Verification items for the finished model (mm, model axes). Face numbers are marked on the shaded views. A direction names the side the tool comes from. Round coordinates to 2 decimals unless told otherwise and drop trailing zeros. Write each loop counter-clockwise with the first axis right and the second up, starting at its lowest first coordinate (ties: lowest second). Pieces come first, ordered by that corner, then holes. Notation, with made-up numbers: (-19, 15.5) - (-3, 15.5) arc R15 ccw to (-3, 21.5) - close; hole circle Ø8 at (49, 11.25). An arc over 180 degrees is marked (long way). Write each question's results on one line, items separated by ' | '.
```python
from build123d import *

# Parameters (mm, degrees)
SKETCH1_W            = 600
SKETCH1_H            = 350
SKETCH1_W_2          = 500
SKETCH1_H_2          = 250
BOSS_EXTRUDE1_DEPTH  = 25
SKETCH2_W            = 50
SKETCH2_H            = 50
BOSS_EXTRUDE2_DEPTH  = 350
SKETCH6_W            = 50
SKETCH6_H            = 25
BOSS_EXTRUDE5_DEPTH  = 300
SKETCH7_W            = 50
SKETCH7_H            = 50
BOSS_EXTRUDE6_DEPTH  = 300
SKETCH8_W            = 50
SKETCH8_H            = 50
BOSS_EXTRUDE7_DEPTH  = 50
SKETCH9_W            = 333.649864746
SKETCH9_H            = 350
SKETCH9_W_2          = 233.483328298
SKETCH9_H_2          = 250
BOSS_EXTRUDE8_DEPTH  = 50
SKETCH10_W           = 50
SKETCH10_H           = 50
BOSS_EXTRUDE10_DEPTH = 10
BOSS_EXTRUDE13_DEPTH = 50
SKETCH15_W           = 30
SKETCH15_H           = 40
CUT_EXTRUDE1_DEPTH   = 50
SKETCH16_R           = 12
CUT_EXTRUDE2_DEPTH   = 50
SKETCH17_W           = 49.023713481
SKETCH17_H           = 36.523713481
CUT_EXTRUDE3_DEPTH   = 100
SKETCH18_W           = 57.595301864
SKETCH18_H           = 39.795828349
CUT_EXTRUDE4_DEPTH   = 100


with BuildPart() as part:
    # Sketch1 → Boss-Extrude1 (new body)
    with BuildSketch(Plane.XY):
        with Locations((250, 125)):
            Rectangle(SKETCH1_W, SKETCH1_H)
        with Locations((250, 125)):
            Rectangle(SKETCH1_W_2, SKETCH1_H_2, mode=Mode.SUBTRACT)
    extrude(amount=BOSS_EXTRUDE1_DEPTH)

    # Sketch2 → Boss-Extrude2 (add)
    with BuildSketch(Plane.XY.offset(25)):
        with Locations((-25, 275)):
            Rectangle(SKETCH2_W, SKETCH2_H)
        with Locations((-25, -25)):
            Rectangle(SKETCH2_W, SKETCH2_H)
    extrude(amount=BOSS_EXTRUDE2_DEPTH)

    # Sketch6 → Boss-Extrude5 (add)
    with BuildSketch(Plane.XZ.offset(-250)):
        with Locations((258.483328298, 12.5)):
            Rectangle(SKETCH6_W, SKETCH6_H)
    extrude(amount=BOSS_EXTRUDE5_DEPTH)

    # Sketch7 → Boss-Extrude6 (add)
    with BuildSketch(Plane.XY.offset(25)):
        with Locations((258.483328298, 119.33659126)):
            Rectangle(SKETCH7_W, SKETCH7_H)
    extrude(amount=BOSS_EXTRUDE6_DEPTH)

    # Sketch8 → Boss-Extrude7 (add)
    with BuildSketch(Plane.XY.offset(325)):
        with Locations((258.483328298, 119.33659126)):
            Rectangle(SKETCH8_W, SKETCH8_H)
    extrude(amount=BOSS_EXTRUDE7_DEPTH)

    # Sketch9 → Boss-Extrude8 (add)
    with BuildSketch(Plane.XY.offset(375)):
        with Locations((116.824932373, 125)):
            Rectangle(SKETCH9_W, SKETCH9_H)
        with Locations((116.741664149, 125)):
            Rectangle(SKETCH9_W_2, SKETCH9_H_2, mode=Mode.SUBTRACT)
    extrude(amount=-BOSS_EXTRUDE8_DEPTH)

    # Sketch10 → Boss-Extrude10 (add)
    with BuildSketch(Plane(origin=(283.483328298, 0, 0), x_dir=(0, 0, -1), z_dir=(1, 0, 0))):
        with Locations((-175, 119.33659126)):
            Rectangle(SKETCH10_W, SKETCH10_H)
    extrude(amount=BOSS_EXTRUDE10_DEPTH)

    # Sketch12 → Boss-Extrude13 (add)
    with BuildSketch(Plane.XZ.offset(-94.33659126)):
        with BuildLine():
            Line((293.483328298, 150), (323.483328298, 150))
            ThreePointArc((323.483328298, 150), (337.625463922, 155.857864376), (343.483328298, 170))
            Line((343.483328298, 170), (343.483328298, 180))
            ThreePointArc((343.483328298, 180), (337.625463922, 194.142135624), (323.483328298, 200))
            Line((323.483328298, 200), (293.483328298, 200))
            Line((293.483328298, 200), (293.483328298, 150))
        make_face()
    extrude(amount=-BOSS_EXTRUDE13_DEPTH)

    # Sketch15 → Cut-Extrude1 (cut)
    with BuildSketch(Plane.XY.offset(200)):
        with Locations((303.483328298, 119.33659126)):
            Rectangle(SKETCH15_W, SKETCH15_H)
    extrude(amount=-CUT_EXTRUDE1_DEPTH, mode=Mode.SUBTRACT)

    # Sketch16 → Cut-Extrude2 (cut)
    with BuildSketch(Plane.XZ.offset(-94.33659126)):
        with Locations(Location((323.483328298, 175, 0), (0, 0, 270))):
            Circle(SKETCH16_R)
    extrude(amount=-CUT_EXTRUDE2_DEPTH, mode=Mode.SUBTRACT)

    # Sketch17 → Cut-Extrude3 (cut)
    with BuildSketch(Plane(origin=(288.483328298, 0, 0), x_dir=(0, 0, -1), z_dir=(1, 0, 0))):
        with Locations((-175.48814326, 119.782326646)):
            Rectangle(SKETCH17_W, SKETCH17_H)
    extrude(amount=CUT_EXTRUDE3_DEPTH, mode=Mode.SUBTRACT)

    # Sketch18 → Cut-Extrude4 (cut)
    with BuildSketch(Plane.XY.offset(200)):
        with Locations((317.28097923, 119.438677086)):
            Rectangle(SKETCH18_W, SKETCH18_H)
    extrude(amount=-CUT_EXTRUDE4_DEPTH, mode=Mode.SUBTRACT)


solid = part.part
```
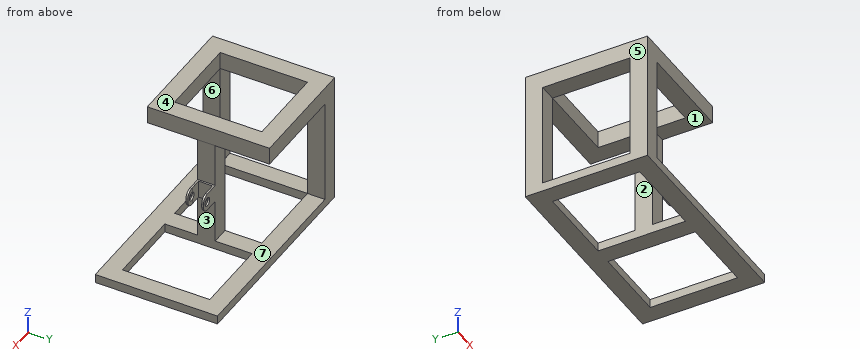
(1) Thickness scan on L1, parallel to Z at x = 254, y = 246.5; L2, parallel to X at y = 141.55, z = 175; L3, parallel to Y at x = 48.5, z = 335.5. Record the ranges inside material, lowest first.
Answer:
L1: 0 to 25, 325 to 375 | L2: 233.48 to 311.48, 335.48 to 343.48 | L3: -50 to 0, 250 to 300
(2) Section check B-B (z = 247.5). Record the cut outline in (x, y), plus the area to 3 significant figures.
Answer:
outline: (-50, -50) - (0, -50) - (0, 0) - (-50, 0) - close; (-50, 250) - (0, 250) - (0, 300) - (-50, 300) - close; (233.48, 94.34) - (283.48, 94.34) - (283.48, 144.34) - (233.48, 144.34) - close | area: 7,500 mm2
(3) Section check A-A (x = 130.5). Record the cut outline in (y, z).
Answer:
outline: (-50, 0) - (0, 0) - (0, 25) - (-50, 25) - close; (-50, 325) - (0, 325) - (0, 375) - (-50, 375) - close; (250, 0) - (300, 0) - (300, 25) - (250, 25) - close; (250, 325) - (300, 325) - (300, 375) - (250, 375) - close
(4) Set-up check for the marked faces 4, 5, 6 and 7: record each of +Z, -Z, +X, -X, +Y, -Y from which the full face is reachable in a straight line by a thin tool's end or side.
Answer:
face 4: +Z, +X, -X, +Y, -Y | face 5: +Z, -Z, -X, +Y, -Y | face 6: +X, +Y, -Y | face 7: +X
(5) Section check D-D (x = 372). Record the cut outline in (y, z).
Answer:
outline: (-50, 0) - (0, 0) - (0, 25) - (-50, 25) - close; (250, 0) - (300, 0) - (300, 25) - (250, 25) - close
(6) Go/stop test with flat-tipped pins: pin 1 Ø15 at (y, z) = (160, 345.5) entering from +X; pin 2 Ø6 at (x, y) = (303, 143.5) entering from +Z; pin 3 Ø3 at (y, z) = (118.5, 84) entering from -X. Record where each tip stops, or that it passes through.
Answer:
pin 1: x = 283.65 | pin 2: z = 200 | pin 3: x = 233.48
(7) Section check C-C (y = 45). Record the cut outline in (x, z).
Answer:
outline: (-50, 0) - (0, 0) - (0, 25) - (-50, 25) - close; (-50, 325) - (0, 325) - (0, 375) - (-50, 375) - close; (233.48, 0) - (283.48, 0) - (283.48, 25) - (233.48, 25) - close; (233.48, 325) - (283.65, 325) - (283.65, 375) - (233.48, 375) - close; (500, 0) - (550, 0) - (550, 25) - (500, 25) - close
(8) Mould release check, pull along Y, two halves, no side actions. Record for the marked faces 1, 2 and 3: released by +Y, released by -Y, zero draft, split by the parting line, or undercut.
Answer:
face 1: zero draft | face 2: undercut | face 3: undercut
